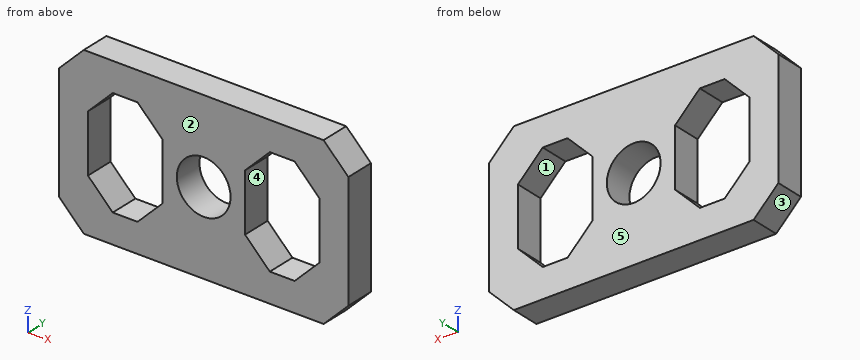
```python
from build123d import *

# Parameters (mm, degrees)
SKETCH1_W           = 70
SKETCH1_H           = 40
SKETCH1_R           = 6.5
SKETCH1_W_2         = 18
SKETCH1_H_2         = 26
BOSS_EXTRUDE1_DEPTH = 7
CHAMFER1_SIZE       = 6


with BuildPart() as part:
    # Sketch1 → Boss-Extrude1 (new body)
    with BuildSketch(Plane(origin=(0, 0, 0), x_dir=(1, 0, 0), z_dir=(0, 1, 0))):
        Rectangle(SKETCH1_W, SKETCH1_H)
        with Locations(Location((0, 0, 0), (0, 0, 270))):
            Circle(SKETCH1_R, mode=Mode.SUBTRACT)
        with Locations((-19, 0)):
            Rectangle(SKETCH1_W_2, SKETCH1_H_2, mode=Mode.SUBTRACT)
        with Locations((19, 0)):
            Rectangle(SKETCH1_W_2, SKETCH1_H_2, mode=Mode.SUBTRACT)
    extrude(amount=BOSS_EXTRUDE1_DEPTH)

    # Chamfer1
    chamfer1_edges = [part.edges().sort_by_distance(p)[0] for p in [
        (-10, 3.5, 13),
        (-10, 3.5, -13),
        (-28, 3.5, -13),
        (-28, 3.5, 13),
        (28, 3.5, 13),
        (28, 3.5, -13),
        (10, 3.5, -13),
        (10, 3.5, 13),
        (35, 3.5, 20),
        (-35, 3.5, 20),
        (-35, 3.5, -20),
        (35, 3.5, -20),
    ]]
    chamfer(chamfer1_edges, length=CHAMFER1_SIZE)


solid = part.part
```
Read the model definition and answer for the solid it produces. Units are mm, in the model's axes. Face numbers are marked on the shaded views. A direction names the side the tool comes from. Coordinates: 2 decimals unless noted, no trailing zeros. Loops run counter-clockwise (first coordinate to the right, second up) from the corner with the lowest first, then second, coordinate; pieces in that order, holes last.
(1) The part is cut by section B-B (x = 25.5). Determine the outline of the cut face in (y, z), and give its area (3 significant figures).
Solution:
outline: (0, -20) - (7, -20) - (7, -9.5) - (0, -9.5) - close; (0, 9.5) - (7, 9.5) - (7, 20) - (0, 20) - close
area: 147 mm2
(2) The part is cut by section D-D (z = -8.5). Determine the outline of the cut face in (x, y), and give its area (3 significant figures).
Solution:
outline: (-35, 0) - (-26.5, 0) - (-26.5, 7) - (-35, 7) - close; (-11.5, 0) - (11.5, 0) - (11.5, 7) - (-11.5, 7) - close; (26.5, 0) - (35, 0) - (35, 7) - (26.5, 7) - close
area: 280 mm2
(3) The mould has two halves that part along X. Classify the marked faces 1, 2 and 3: released by +X, released by -X, zero draft, split by the parting line, or undercut.
Solution:
face 1: undercut
face 2: zero draft
face 3: released by -X
(4) The part is cut by section A-A (z = 0). Determine the outline of the cut face in (x, y), and give its area (3 significant figures).
Solution:
outline: (-35, 0) - (-28, 0) - (-28, 7) - (-35, 7) - close; (-10, 0) - (-6.5, 0) - (-6.5, 7) - (-10, 7) - close; (6.5, 0) - (10, 0) - (10, 7) - (6.5, 7) - close; (28, 0) - (35, 0) - (35, 7) - (28, 7) - close
area: 147 mm2
(5) A tool of negligible diameter and unlimited length cuts with its end or side. For the marked faces 4 and 5, from which of +Z, -Z, +X, -X, +Y, -Y can it reach the whole face along a straight path? Write none if from no direction.
Solution:
face 4: +Y, -Y
face 5: +Z, -Z, +X, -X, +Y
(6) The part is cut by section C-C (y = 3). Determine the outline of the cut face in (x, z), and give its area (3 significant figures).
Solution:
outline: (-35, -14) - (-29, -20) - (29, -20) - (35, -14) - (35, 14) - (29, 20) - (-29, 20) - (-35, 14) - close; hole (-28, -7) - (-22, -13) - (-16, -13) - (-10, -7) - (-10, 7) - (-16, 13) - (-22, 13) - (-28, 7) - close; hole circle Ø13 at (0, 0); hole (10, -7) - (16, -13) - (22, -13) - (28, -7) - (28, 7) - (22, 13) - (16, 13) - (10, 7) - close
area: 1,800 mm2
(7) Consider line 1 along X through (y, z) = (3, 0); line 2 along X through (y, z) = (6.75, -12); line 3 along X through (y, z) = (4, 2.5). Determine where each line is inside the solid, lowest interval first.
Solution:
line 1: x = -35 to -28, -10 to -6.5, 6.5 to 10, 28 to 35
line 2: x = -35 to -23, -15 to 15, 23 to 35
line 3: x = -35 to -28, -10 to -6, 6 to 10, 28 to 35
